Geometry: see drawing. Coordinates: mm, zero at the bounding-box minimum. Give positions to 0.01 mm unless a question says otherwise; leave off trailing zeros. Write each loop counter-clockwise with the first axis right and the second up, starting at its lowest first coordinate (ties: lowest second). Pieces come first, ordered by that corner, then holes. Notation, with made-up numbers: M 57,5.25 L 65,5.25 A21 ccw 65,17.25 Z; hole C -1,41.5 d11. An arc over 180 degrees is marked long. Use a Markdown table: item, result. Add a question column.
1) Section B-B on z = 8. Return the cut outline in (x, y).
2) Section C-C on y = 0.4. State how many separate pieces and enclosed holes the cut face has, then the cut area to 3 significant figures.
3) Line query: line 1 (X direction, y = 0.15, z = 10.25); line 2 (Z direction, x = 15.5, y = 0.4); line 3 (Z direction, x = 8, y = 0.5). Output: solid intervals per line, ascending.
4) Section A-A on x = 15.5. Return the cut outline in (y, z).
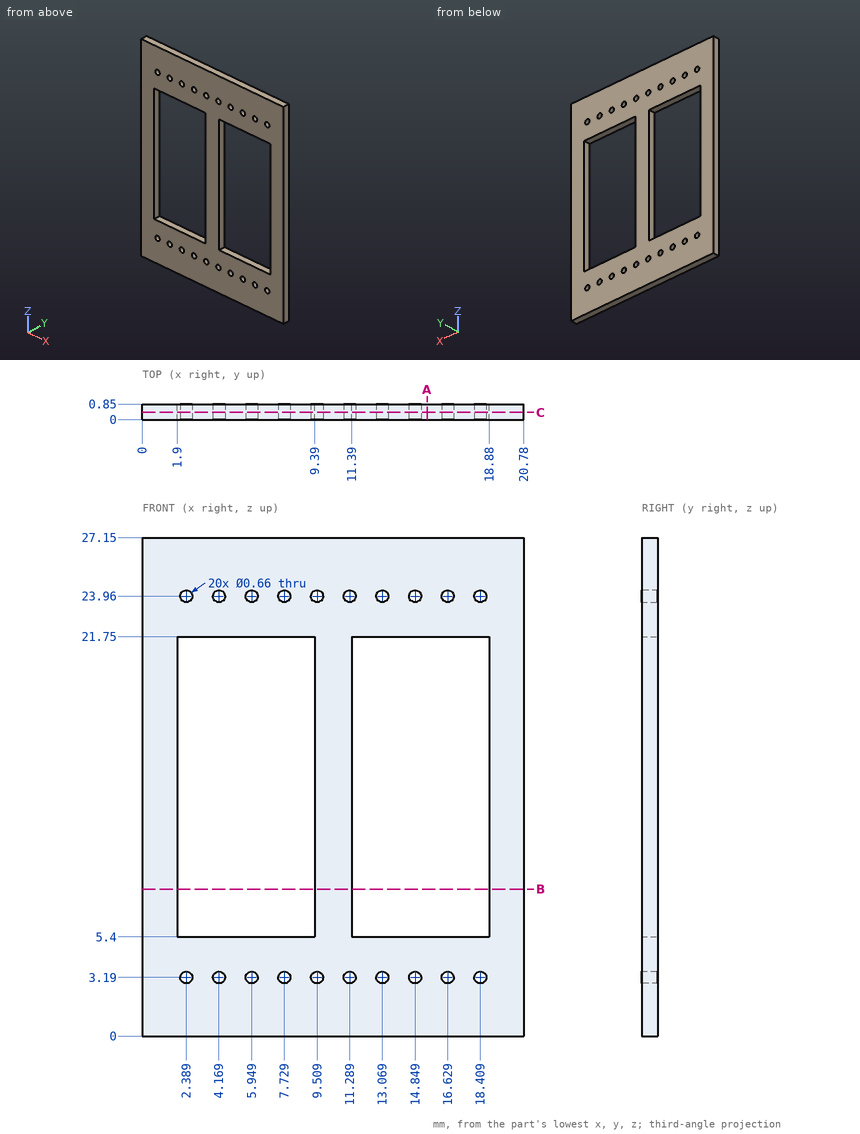
Found:
| question | item | result |
|---|---|---|
| 1 | outline | M 0,0 L 1.9,0 L 1.9,0.85 L 0,0.85 Z; M 9.39,0 L 11.39,0 L 11.39,0.85 L 9.39,0.85 Z; M 18.88,0 L 20.78,0 L 20.78,0.85 L 18.88,0.85 Z |
| 2 | separate pieces | 1 |
| 2 | enclosed holes | 22 |
| 2 | area | 312 mm² |
| 3 | line 1 | 0 to 1.9, 9.39 to 11.39, 18.88 to 20.78 |
| 3 | line 2 | 0 to 5.4, 21.75 to 27.15 |
| 3 | line 3 | 0 to 3, 3.38 to 5.4, 21.75 to 23.77, 24.15 to 27.15 |
| 4 | outline | M 0,0 L 0.85,0 L 0.85,5.4 L 0,5.4 Z; M 0,21.75 L 0.85,21.75 L 0.85,27.15 L 0,27.15 Z |
